Autodesk Inventor part; units mm, degrees
ref_plane "YZ Plane" through (0, 0, 0) normal (1, 0, 0) x (0, 1, 0)
ref_plane "XZ Plane" through (0, 0, 0) normal (0, 1, 0) x (-1, 0, 0)
ref_plane "XY Plane" through (0, 0, 0) normal (0, 0, 1) x (1, 0, 0)
sketch "Esboço1" plane through (0, 0, 0) normal (0, 0, 1) x (1, 0, 0)
  line L0 (-300, -150) -> (300, -150)
  line L1 (300, -150) -> (300, 150)
  line L2 (300, 150) -> (-300, 150)
  line L3 (-300, 150) -> (-300, -150)
  line L4 (-300, -150) -> (300, 150) construction
  line L5 (300, -150) -> (-300, 150) construction
  circle A0 centre (0, 0) radius 45
  dimension "d0" = 600
  dimension "d1" = 300
  dimension "d2" = 90
extrude "Extrusão1" add sketch "Esboço1" along normal blind 8
sketch "Esboço2" plane through (0, 0, 8) normal (0, 0, 1) x (1, 0, 0)
  line L0 (-250, -146) -> (250, 146) construction
  line L1 (250, -146) -> (-250, 146) construction
  circle A0 centre (-250, 146) radius 2
  circle A1 centre (0, 146) radius 2
  circle A2 centre (250, 146) radius 2
  circle A3 centre (250, -146) radius 2
  circle A4 centre (0, -146) radius 2
  circle A5 centre (-250, -146) radius 2
  point P0 (0, 0)
  dimension "d5" = 292
  dimension "d7" = 4
  dimension "d8" = 4
  dimension "d9" = 4
  dimension "d10" = 4
  dimension "d11" = 4
  dimension "d12" = 4
extrude "Extrusão2" cut sketch "Esboço2" against normal blind 10
chamfer "Chanfro1" distance 1 angle 45 6 edges at (-252, 146, 8) (-2, 146, 8) (248, 146, 8) (248, -146, 8) (-2, -146, 8) (-252, -146, 8)
properties part number "base-inferior"
Model file for the job. Use its own axes, mm. Coordinates: 2 decimals unless noted, no trailing zeros. Loops run counter-clockwise (first coordinate to the right, second up) from the corner with the lowest first, then second, coordinate; pieces in that order, holes last. Notation, with made-up numbers: (-8, -24.75) - (8, -24.75) arc R23 cw to (8, 2.25) - close; hole circle Ø1 at (-9.75, -0.75). An arc over 180 degrees is marked (long way). Answer as a JSON object with one key per item and string values. Group by question number.
(1) Cut at B-B (y = 0). Give the cut face in (x, z).
(2) Cut at C-C (x = -33). Give the cut face in (y, z).
(3) Flat gauge pins, fed straight in: pin 1 (3.5 mm diameter, centred on x = 250, y = 146, fed in from -Z); pin 2 (1 mm diameter, centred on x = 3.5, y = 107, fed in from -Z); pin 3 (5 mm diameter, centred on x = -250, y = 146, fed in from +Z). Where does each tip first touch, or does it go through?
(4) Probe line 1 along Y through (x, z) = (0, 4.5); line 2 along X through (y, z) = (146, 2.5); line 3 along Y through (x, z) = (-250, 1.5). List the from-to ranges inside material, lowest first.
(5) Two-plate mould, pull along Y, no slides. Class faces 1 (the face through (20.765, 39.923, 3.944)), 2 (the face through (-4, -65, 0)): released by +Y, released by -Y, zero draft, split by the parting line, or undercut.
(6) Cut at A-A (z = 1.5). Give the cut face in (x, y).
Geometry says:
{
 "1": {"outline": "(-300, 0) - (-45, 0) - (-45, 8) - (-300, 8) - close; (45, 0) - (300, 0) - (300, 8) - (45, 8) - close"},
 "2": {"outline": "(-150, 0) - (-30.59, 0) - (-30.59, 8) - (-150, 8) - close; (30.59, 0) - (150, 0) - (150, 8) - (30.59, 8) - close"},
 "3": {"pin 1": "passes through", "pin 2": "stops at z = 0", "pin 3": "stops at z = 7.5"},
 "4": {"line 1": "y = -150 to -148, -144 to -45, 45 to 144, 148 to 150", "line 2": "x = -300 to -252, -248 to -2, 2 to 248, 252 to 300", "line 3": "y = -150 to -148, -144 to 144, 148 to 150"},
 "5": {"face 1": "undercut", "face 2": "zero draft"},
 "6": {"outline": "(-300, -150) - (300, -150) - (300, 150) - (-300, 150) - close; hole circle Ø4 at (-250, -146); hole circle Ø4 at (-250, 146); hole circle Ø90 at (0, 0); hole circle Ø4 at (0, -146); hole circle Ø4 at (0, 146); hole circle Ø4 at (250, -146); hole circle Ø4 at (250, 146)"}
}
